```python
from build123d import *

# Parameters (mm, degrees)
SKETCH1_R           = 20
BOSS_EXTRUDE1_DEPTH = 10
SKETCH2_R           = 2.5
SKETCH2_R_2         = 2.302418505
CUT_EXTRUDE1_DEPTH  = 35
CUT_EXTRUDE2_START  = -1
CUT_EXTRUDE2_DEPTH  = 1


with BuildPart() as part:
    # Sketch1 → Boss-Extrude1 (new body)
    with BuildSketch(Plane.XY):
        Circle(SKETCH1_R)
    extrude(amount=BOSS_EXTRUDE1_DEPTH)

    # Sketch2 → Cut-Extrude1 (cut)
    with BuildSketch(Plane.XY.offset(10)):
        with Locations((-15, 0)):
            Circle(SKETCH2_R)
        with Locations((-11.490666647, 9.641814145)):
            Circle(SKETCH2_R)
        with Locations((-2.604722665, 14.772116295)):
            Circle(SKETCH2_R)
        with Locations((7.5, 12.990381057)):
            Circle(SKETCH2_R)
        with Locations((14.095389312, 5.13030215)):
            Circle(SKETCH2_R)
        with Locations((14.095389312, -5.13030215)):
            Circle(SKETCH2_R)
        with Locations((7.5, -12.990381057)):
            Circle(SKETCH2_R)
        with Locations((-2.604722665, -14.772116295)):
            Circle(SKETCH2_R)
        with Locations((-11.490666647, -9.641814145)):
            Circle(SKETCH2_R)
        with Locations((-5.106965508, 4.285252874)):
            Circle(SKETCH2_R_2)
        with Locations((6.264620604, 2.280135429)):
            Circle(SKETCH2_R_2)
        with Locations((-1.157655097, -6.565388303)):
            Circle(SKETCH2_R_2)
    extrude(amount=-CUT_EXTRUDE1_DEPTH, mode=Mode.SUBTRACT)

    # Sketch3 → Cut-Extrude2 (cut)
    with BuildSketch(Plane.XY.offset(10).offset(CUT_EXTRUDE2_START)):
        with BuildLine():
            ThreePointArc((-18.958988491, -6.368418596), (-18.793852416, -6.840402867), (-18.616968347, -7.308111217))
            Line((-18.616968347, -7.308111217), (-0.100255822, -0.568579021))
            Line((-0.100255822, -0.568579021), (14.994706531, -13.234756365))
            ThreePointArc((14.994706531, -13.234756365), (15.320888862, -12.855752194), (15.637494141, -12.468711922))
            Line((15.637494141, -12.468711922), (0.542531788, 0.197465422))
            Line((0.542531788, 0.197465422), (3.964281959, 19.603174961))
            ThreePointArc((3.964281959, 19.603174961), (3.472963553, 19.69615506), (2.979474206, 19.776823139))
            Line((2.979474206, 19.776823139), (-0.442275965, 0.371113599))
            Line((-0.442275965, 0.371113599), (-18.958988491, -6.368418596))
        make_face()
    cut_extrude2 = extrude(amount=CUT_EXTRUDE2_DEPTH, mode=Mode.SUBTRACT)

    # Mirror1: Cut-Extrude2 across plane
    add(cut_extrude2.mirror(Plane(origin=(0, 0, 5), x_dir=(1, 0, 0), z_dir=(0, 0, -1))), mode=Mode.SUBTRACT)


solid = part.part
```
Check sheet for the modelled part. Datum: model origin and axes. Units: mm. A direction names the side the tool comes from. Round coordinates to 2 decimals unless told otherwise and drop trailing zeros. Order: outer loops, then holes, each group sorted by start corner. A loop starts at its lowest first (then second) coordinate and runs counter-clockwise, first axis right, second up. Notation, with made-up numbers: (52, -8.75) -> (66, -8.75) arc R18 cw to (66, 1.25) -> close; hole circle Ø2 at (49.5, -17.75). An arc over 180 degrees is marked (long way). One line per item, written item: value. Start each with the question number.
Q1. Set-up check for faces 1 (the face through (2.23, 9.76, 0.51)), 2 (the face through (2.23, 9.76, 9.49)), 3 (the face through (-13.475, -11.163, 5.07)): record each of +Z, -Z, +X, -X, +Y, -Y from which the full face is reachable in a straight line by a thin tool's end or side.
Q2. Gauge pin test, flat ends, axial feed: pin 1 Ø4 at (x, y) = (14.1, 5.13) entering from -Z; pin 2 Ø6 at (y, z) = (5, 5.5) entering from +X; pin 3 Ø1 at (x, z) = (13, 6.5) entering from +Y; pin 4 Ø5 at (x, z) = (-16, 7) entering from -Y. Record the tip position at first contact, or that the pin passes through.
Q3. Cross-section at C-C (x = 7.5). Record the boundary of the cut face in (y, z), and give its area (3 significant figures).
Q4. Thickness scan on line 1 (X direction, y = -14.5, z = 2.25); line 2 (X direction, y = 8.5, z = 0.75); line 3 (Y direction, x = 15, z = 3). Record the ranges inside material, lowest first.
Q5. Mould release check, pull along X, two halves, no side actions. Record for faces 4 (the face through (7.34, -6.81, 0.51)), 5 (the face through (-9, 7, 0)): pulls with the +X half, pulls with the -X half, needs draft (parallel to the pull), parting line crosses it, or undercut.
Q6. Cross-section at D-D (z = 4). Give the number of separate pieces and of enclosed holes in the cut face, and give its area (3 significant figures).
Q7. Cross-section at B-B (y = -16). Record the boundary of the cut face in (x, z).
Q8. Cross-section at A-A (x = -15). Record the boundary of the cut face in (y, z), and give its area (3 significant figures).
Completed:
1. face 1: -Z
1. face 2: +Z
1. face 3: +Z, -Z
2. pin 1: passes through
2. pin 2: stops at x = 19.9
2. pin 3: stops at y = 15.61
2. pin 4: stops at y = -14.76
3. outline: (-18.54, 0) -> (-15.49, 0) -> (-15.49, 10) -> (-18.54, 10) -> close; (-10.49, 0) -> (-6.95, 0) -> (-6.95, 1) -> (-5.64, 1) -> (-5.64, 0) -> (0.34, 0) -> (0.34, 10) -> (-5.64, 10) -> (-5.64, 9) -> (-6.95, 9) -> (-6.95, 10) -> (-10.49, 10) -> close; (4.22, 0) -> (10.49, 0) -> (10.49, 10) -> (4.22, 10) -> close; (15.49, 0) -> (18.54, 0) -> (18.54, 10) -> (15.49, 10) -> close
3. area: 229 mm²
4. line 1: x = -13.77 to -5.09, -0.12 to 5.51, 9.49 to 13.77
4. line 2: x = -18.1 to -13.71, -9.27 to 0.99, 2.01 to 18.1
4. line 3: y = -13.23 to -7.46, -2.8 to 2.8, 7.46 to 13.23
5. face 4: undercut
5. face 5: needs draft
6. separate pieces: 1
6. enclosed holes: 12
6. area: 1,030 mm²
7. outline: (-12, 0) -> (-4.78, 0) -> (-4.78, 10) -> (-12, 10) -> close; (-0.43, 0) -> (12, 0) -> (12, 10) -> (-0.43, 10) -> close
8. outline: (-13.23, 0) -> (-5.99, 0) -> (-5.99, 1) -> (-4.93, 1) -> (-4.93, 0) -> (-2.5, 0) -> (-2.5, 10) -> (-4.93, 10) -> (-4.93, 9) -> (-5.99, 9) -> (-5.99, 10) -> (-13.23, 10) -> close; (2.5, 0) -> (13.23, 0) -> (13.23, 10) -> (2.5, 10) -> close
8. area: 212 mm²
